The listing builds one solid part. Answer for the finished solid, in the listing's coordinates (mm). A direction names the side the tool comes from. Give positions to 0.01 mm unless a question says otherwise; leave off trailing zeros. Write each loop counter-clockwise with the first axis right and the second up, starting at its lowest first coordinate (ties: lowest second). Pieces come first, ordered by that corner, then holes. Notation, with made-up numbers: (83.25, 84) -> (140.25, 84) arc R34 ccw to (140.25, 116) -> close; hole circle Ø2 at (83, 75). An arc over 180 degrees is marked (long way). Put each result on its own line as item: value. Start each with the question number.
1) A cutting plane is placed at C-C (z = -5.25). Write down the section's boundary in (x, y), then the cut area to 3 significant figures.
2) A cutting plane is placed at A-A (y = 0.2). Write down the section's boundary in (x, z), then the cut area to 3 significant figures.
3) A cutting plane is placed at D-D (y = 0.95). Write down the section's boundary in (x, z).
4) Flat-ended cylindrical pins translate along their axes: pin 1 Ø0.5 at (x, z) = (4, -6) entering from +Y; pin 2 Ø3 at (x, z) = (4, -3.75) entering from -Y; pin 3 Ø3.5 at (x, z) = (5.5, -3.5) entering from -Y. Find the tip coordinate at first contact, or state that the pin passes through.
5) For a pull along Z with two mould halves and no side action, classify faces 1 (the flat face through (4, 2.6, -3)), 2 (the cylindrical face through (6.51, -1.48, -7.51)), 3 (the flat face through (4, -1, -8)) as released by +Z, released by -Z, zero draft, split by the parting line, or undercut.
6) Find the intervals of material crossed by line 1 along Y through (x, z) = (1.5, -6.5); line 2 along Z through (x, y) = (2.75, -0.05); line 3 along Y through (x, z) = (4.75, -4), in increasing order. Write a range as from..to.
7) For faces 4 (the cylindrical face through (2.94, 0.2, -2.36)), 5 (the flat face through (4, 2.6, -6)), 6 (the flat face through (4, 3, -4)), 7 (the flat face through (4, -1, -7)), determine the directions among +Z, -Z, +X, -X, +Y, -Y from which every point of the face is accessible in a straight line to the end or side of a thin tool.
8) A cutting plane is placed at B-B (x = 3). Write down the section's boundary in (y, z).
from build123d import *

# Parameters (mm, degrees)
SKETCH1_W               = 8
SKETCH1_H               = 8
BOSS_EXTRUDE1_DEPTH     = 3
CUT_EXTRUDE1_DEPTH      = 12.704699911
CUT_EXTRUDE1_DEPTH_BACK = 12.704699911
CUT_EXTRUDE2_DEPTH      = 11
SKETCH4_R               = 1.75
CUT_EXTRUDE3_DEPTH      = 0.4
SKETCH5_W               = 8
SKETCH5_H               = 1
BOSS_EXTRUDE2_DEPTH     = 2
FILLET1_R               = 4
SKETCH6_W               = 0.961538461
SKETCH6_H               = 0.961538462
CUT_EXTRUDE4_DEPTH      = 0.4


with BuildPart() as part:
    # Sketch1 → Boss-Extrude1 (new body)
    with BuildSketch(Plane(origin=(0, 0, 0), x_dir=(1, 0, 0), z_dir=(0, 1, 0))):
        with Locations((4, 4)):
            Rectangle(SKETCH1_W, SKETCH1_H)
    extrude(amount=BOSS_EXTRUDE1_DEPTH)

    # Sketch2 → Cut-Extrude1 (cut, two sides: drawn at the far end of the back side and taken through both)
    with BuildSketch(Plane.XY.offset(-CUT_EXTRUDE1_DEPTH_BACK)):
        Polygon((0, 0), (0.6, 3), (0, 3), align=None)
        Polygon((8, 0), (7.4, 3), (8, 3), align=None)
    extrude(amount=CUT_EXTRUDE1_DEPTH + CUT_EXTRUDE1_DEPTH_BACK, mode=Mode.SUBTRACT)

    # Sketch3 → Cut-Extrude2 (cut)
    with BuildSketch(Plane(origin=(0, 0, 0), x_dir=(0, 0, -1), z_dir=(1, 0, 0))):
        Polygon((0, 0), (0.6, 3), (0, 3), align=None)
        Polygon((8, 3), (7.4, 3), (8, 0), align=None)
    extrude(amount=CUT_EXTRUDE2_DEPTH, mode=Mode.SUBTRACT)

    # Sketch4 → Cut-Extrude3 (cut)
    with BuildSketch(Plane.XZ):
        with Locations(Location((4, -3.75, 0), (0, 0, 270))):
            Circle(SKETCH4_R)
    extrude(amount=-CUT_EXTRUDE3_DEPTH, mode=Mode.SUBTRACT)

    # Sketch5 → Boss-Extrude2 (add)
    with BuildSketch(Plane.XZ):
        with Locations((4, -7.5)):
            Rectangle(SKETCH5_W, SKETCH5_H)
    extrude(amount=BOSS_EXTRUDE2_DEPTH)

    # Fillet1
    # the kernel refuses this fillet: 4 mm, written as the material it takes off along each edge
    with BuildSketch(Plane(origin=(8, -2, -16.660254038), x_dir=(0, 1, 0), z_dir=(0, 0, 1)), Plane(origin=(0, -2, 1.660254038), x_dir=(0, 1, 0), z_dir=(0, 0, -1))) as fillet1_piece_1:
        with BuildLine():
            CenterArc((4, 3.464101615), FILLET1_R, 180, 60)
            Line((0, 3.464101615), (-0.08, 3.464101615))
            Line((-0.08, 3.464101615), (-0.08, 0))
            Line((-0.08, 0), (0, -0.08))
            ThreePointArc((0, -0.08), (1, -0.08), (1.96, -0.069282032))
            Line((1.96, -0.069282032), (2, 0))
        make_face()
    extrude(amount=18.320508076, mode=Mode.SUBTRACT)

    # Sketch6 → Cut-Extrude4 (cut)
    with BuildSketch(Plane(origin=(0, 3, 0), x_dir=(1, 0, 0), z_dir=(0, 1, 0))):
        with Locations((4.106375193, 5.877622732)):
            Rectangle(SKETCH6_W, SKETCH6_H)
        with BuildLine():
            Line((3.625605963, 3.666084271), (4.587144424, 3.666084271))
            Line((4.587144424, 3.666084271), (4.587144424, 2.966965681))
            add(Edge.make_bspline(
                [(4.587144424, 2.966965681), (4.586700802, 2.899821455), (4.585863185, 2.773044347), (4.571180714, 2.594207821), (4.550779556, 2.437158718), (4.518324342, 2.299878361), (4.47486997, 2.175902827), (4.413432502, 2.062461013), (4.337876173, 1.953901165), (4.245458326, 1.85350819), (4.139144335, 1.760654771), (4.017702284, 1.679908688), (3.88401418, 1.607967915), (3.787969656, 1.570094118), (3.738787052, 1.550699655)],
                knots=[0, 0, 0, 0, 1.347156832, 2.543608823, 3.599300285, 4.522475688, 5.370350604, 6.227678973, 7.103274953, 8.018757603, 8.959280198, 9.929437417, 10.939703653, 12, 12, 12, 12], degree=3))
            Line((3.738787052, 1.550699655), (3.561503399, 1.93531504))
            add(Edge.make_bspline(
                [(3.561503399, 1.93531504), (3.604439047, 1.952873279), (3.686527672, 1.986442858), (3.795938691, 2.052543314), (3.885105421, 2.129792439), (3.955780801, 2.218165676), (4.006656804, 2.32038588), (4.045456087, 2.435104657), (4.0674697, 2.56519407), (4.07197182, 2.656725854), (4.074323911, 2.704545809)],
                knots=[0, 0, 0, 0, 1.115416734, 2.132564161, 3.06091458, 3.941973359, 4.836922823, 5.794989041, 6.848011894, 8, 8, 8, 8], degree=3))
            Line((4.074323911, 2.704545809), (3.625605963, 2.704545809))
            Line((3.625605963, 2.704545809), (3.625605963, 3.666084271))
        make_face()
    extrude(amount=-CUT_EXTRUDE4_DEPTH, mode=Mode.SUBTRACT)


solid = part.part
Reply:
1. outline: (0, 0) -> (3.1, 0) -> (3.1, 0.4) -> (4.9, 0.4) -> (4.9, 0) -> (8, 0) -> (7.4, 3) -> (0.6, 3) -> close
1. area: 21.5 mm2
2. outline: (0.04, -7.96) -> (7.96, -7.96) -> (7.96, -0.04) -> (0.04, -0.04) -> close; hole circle Ø3.5 at (4, -3.75)
2. area: 53.1 mm2
3. outline: (0.19, -7.81) -> (7.81, -7.81) -> (7.81, -0.19) -> (0.19, -0.19) -> close
4. pin 1: stops at y = 2.6
4. pin 2: stops at y = 0.4
4. pin 3: stops at y = 0
5. face 1: undercut
5. face 2: zero draft
5. face 3: released by -Z
6. line 1: y = 0..3
6. line 2: z = -8..-7
6. line 3: y = 0.4..3
7. face 4: -Y
7. face 5: +Y
7. face 6: +Z, -Z, +X, -X, +Y
7. face 7: +Z, +X, -X, -Y
8. outline: (-1.97, -8) -> (0, -8) -> (3, -7.4) -> (3, -0.6) -> (0, 0) -> (0, -2.31) -> (0.4, -2.31) -> (0.4, -5.19) -> (0, -5.19) -> (0, -7) -> (-1.97, -7) -> close
